Input: part model. Units: mm. Frame: model coordinates. Coordinates: 2 decimals unless noted, no trailing zeros. Write each loop counter-clockwise with the first axis right and the second up, starting at its lowest first coordinate (ties: lowest second). Pieces come first, ordered by that corner, then holes. Notation, with made-up numbers: M 66.5,51.25 L 112.5,51.25 A19 ccw 112.5,63.25 Z; hole C 42.5,-23 d9. An arc over 180 degrees is marked long. Use one line per item in the form item = value.
Autodesk Inventor part; units mm, degrees
ref_plane "YZ Plane" through (0, 0, 0) normal (1, 0, 0) x (0, 1, 0)
ref_plane "XZ Plane" through (0, 0, 0) normal (0, 1, 0) x (-1, 0, 0)
ref_plane "XY Plane" through (0, 0, 0) normal (0, 0, 1) x (1, 0, 0)
sketch "Sketch1" plane through (0, 0, 0) normal (0, 0, 1) x (1, 0, 0)
  line L0 (0, 0) -> (10.3, 0)
  line L1 (10.3, 0) -> (10.3, 14.5)
  line L2 (10.3, 14.5) -> (0, 14.5)
  line L3 (0, 14.5) -> (0, 0)
  line L4 (3.9, 0) -> (6.4, 0)
  line L5 (6.4, 0) -> (6.4, 14.5)
  line L6 (6.4, 14.5) -> (3.9, 14.5)
  line L7 (3.9, 14.5) -> (3.9, 0)
  line L8 (0, 0) -> (10.3, 0)
  line L9 (10.3, 0) -> (10.3, -3)
  line L10 (10.3, -3) -> (0, -3)
  line L11 (0, -3) -> (0, 0)
  circle A0 centre (1.95, 7.25) radius 1.15
  circle A1 centre (8.35, 7.25) radius 1.15
  dimension "d0" = 10.3
  dimension "d1" = 14.5
  dimension "d2" = 2.5
  dimension "d3" = 3
  dimension "d4" = 3.9
  dimension "d5" = 0
  dimension "d6" = 2.3
  dimension "d7" = 1.95
  dimension "d8" = 7.25
  dimension "d9" = 2.3
  dimension "d10" = 1.95
  dimension "d11" = 7.25
extrude "Extrusion2" add sketch "Sketch1" along normal blind 1 contours L3 L2 L7 L0 | L7 L2 L5 L0 | L5 L2 L1 L0
equation "\"d4\" = -0.5 * d2 + 0.5 * d0"
equation "\"d7\" = 0.5 * d4"
equation "\"d8\" = 0.5 * d1"
equation "\"d9\" = d6"
equation "\"d10\" = d7"
equation "\"d11\" = d8"
properties part number "control_arm_backplate_mount"
(1) Section query D-D on x = 7.75. Return the cut outline in (y, z).
Computed:
outline = M 0,0 L 6.27,0 L 6.27,1 L 0,1 Z; M 8.23,0 L 14.5,0 L 14.5,1 L 8.23,1 Z
(2) Pull-direction query (X, two-part tool) for faces 1 (the cylindrical face through (1.8, 6.11, 0.49)), 2 (the flat face through (10.3, 7.1, 0.5)), 3 (the cylindrical face through (8.2, 6.11, 0.49)), 4 (the flat face through (5, 7, 0)); classes: pulls with the +X half, pulls with the -X half, needs draft (parallel to the pull), parting line crosses it, or undercut.
Computed:
face_1 = undercut
face_2 = pulls with the +X half
face_3 = undercut
face_4 = needs draft
(3) Line query: probe 1 along Y at (x, z) = (1.95, 0.75); probe 2 along Y at (x, z) = (2.5, 0.2). Output: solid intervals per line, ascending.
Computed:
probe_1 = 0 to 6.1, 8.4 to 14.5
probe_2 = 0 to 6.24, 8.26 to 14.5
(4) Section query B-B on y = 7.25. Return the cut outline in (x, z), plus the area to 3 significant figures.
Computed:
outline = M 0,0 L 0.8,0 L 0.8,1 L 0,1 Z; M 3.1,0 L 7.2,0 L 7.2,1 L 3.1,1 Z; M 9.5,0 L 10.3,0 L 10.3,1 L 9.5,1 Z
area = 5.70 mm^2
(5) Section query A-A on x = 1.95. Return the cut outline in (y, z).
Computed:
outline = M 0,0 L 6.1,0 L 6.1,1 L 0,1 Z; M 8.4,0 L 14.5,0 L 14.5,1 L 8.4,1 Z
(6) Section query C-C on z = 0.3. Return the cut outline in (x, y), plus the area to 3 significant figures.
Computed:
outline = M 0,0 L 10.3,0 L 10.3,14.5 L 0,14.5 Z; hole C 1.95,7.25 d2.3; hole C 8.35,7.25 d2.3
area = 141 mm^2
